Read the model definition and answer for the solid it produces. Units are mm, in the model's axes. A direction names the side the tool comes from. Coordinates: 2 decimals unless noted, no trailing zeros. Loops run counter-clockwise (first coordinate to the right, second up) from the corner with the lowest first, then second, coordinate; pieces in that order, holes last. Notation, with made-up numbers: (47.5, -28.5) - (81.5, -28.5) arc R6 ccw to (81.5, -20.5) - close; hole circle Ø9 at (82.5, 69). An arc over 180 degrees is marked (long way). One line per item, written item: value. Start each with the question number.
from build123d import *

# Parameters (mm, degrees)
SKETCH1_W           = 66.5
SKETCH1_H           = 180
BOSS_EXTRUDE1_DEPTH = 180
SKETCH3_W           = 160
SKETCH3_H           = 160
CUT_EXTRUDE1_DEPTH  = 180
SKETCH8_W           = 66.5
SKETCH8_H           = 40
BOSS_EXTRUDE2_DEPTH = 5
SKETCH10_W          = 66.5
SKETCH10_H          = 40
BOSS_EXTRUDE3_DEPTH = 5
SKETCH5_R           = 14
CUT_EXTRUDE3_DEPTH  = 10
SKETCH7_R           = 14
CUT_EXTRUDE4_DEPTH  = 10
CUT_EXTRUDE5_DEPTH  = 5
CUT_EXTRUDE6_START  = -5
CUT_EXTRUDE6_DEPTH  = 5
SKETCH12_W          = 66.5
SKETCH12_H          = 40
BOSS_EXTRUDE8_DEPTH = 5
SKETCH15_R          = 14
CUT_EXTRUDE7_DEPTH  = 200
SKETCH16_W          = 66.5
SKETCH16_H          = 40
BOSS_EXTRUDE9_DEPTH = 5
FILLET1_R           = 10
FILLET2_R           = 10


with BuildPart() as part:
    # Sketch1 → Boss-Extrude1 (new body)
    with BuildSketch(Plane.XY):
        with Locations((33.25, 90)):
            Rectangle(SKETCH1_W, SKETCH1_H)
    extrude(amount=BOSS_EXTRUDE1_DEPTH)

    # Sketch3 → Cut-Extrude1 (cut)
    with BuildSketch(Plane.ZY):
        with Locations((90, 90)):
            Rectangle(SKETCH3_W, SKETCH3_H)
    extrude(amount=-CUT_EXTRUDE1_DEPTH, mode=Mode.SUBTRACT)

    # Sketch8 → Boss-Extrude2 (add)
    with BuildSketch(Plane.XY.offset(10)):
        with Locations((33.25, 150)):
            Rectangle(SKETCH8_W, SKETCH8_H)
    extrude(amount=BOSS_EXTRUDE2_DEPTH)

    # Sketch10 → Boss-Extrude3 (add)
    with BuildSketch(Plane(origin=(0, 0, 170), x_dir=(-1, 0, 0), z_dir=(0, 0, -1))):
        with Locations((-33.25, 150)):
            Rectangle(SKETCH10_W, SKETCH10_H)
    extrude(amount=BOSS_EXTRUDE3_DEPTH)

    # Sketch5 → Cut-Extrude3 (cut)
    with BuildSketch(Plane(origin=(0, 180, 0), x_dir=(1, 0, 0), z_dir=(0, 1, 0))):
        with Locations(Location((49.5, -90, 0), (0, 0, 270))):
            Circle(SKETCH5_R)
    extrude(amount=-CUT_EXTRUDE3_DEPTH, mode=Mode.SUBTRACT)

    # Sketch7 → Cut-Extrude4 (cut)
    with BuildSketch(Plane.XZ):
        with Locations(Location((49.5, 50, 0), (0, 0, 270))):
            Circle(SKETCH7_R)
        with Locations(Location((49.5, 130, 0), (0, 0, 270))):
            Circle(SKETCH7_R)
    extrude(amount=-CUT_EXTRUDE4_DEPTH, mode=Mode.SUBTRACT)

    # Sketch9 → Cut-Extrude5 (cut)
    with BuildSketch(Plane.XY.offset(15)):
        with BuildLine():
            Line((60.5, 164.5), (7.5, 164.5))
            ThreePointArc((7.5, 164.5), (5.378679656, 163.621320344), (4.5, 161.5))
            Line((4.5, 161.5), (4.5, 138.5))
            ThreePointArc((4.5, 138.5), (5.378679656, 136.378679656), (7.5, 135.5))
            Line((7.5, 135.5), (60.5, 135.5))
            ThreePointArc((60.5, 135.5), (62.621320344, 136.378679656), (63.5, 138.5))
            Line((63.5, 138.5), (63.5, 161.5))
            ThreePointArc((63.5, 161.5), (62.621320344, 163.621320344), (60.5, 164.5))
        make_face()
    extrude(amount=-CUT_EXTRUDE5_DEPTH, mode=Mode.SUBTRACT)

    # Sketch11 → Cut-Extrude6 (cut)
    with BuildSketch(Plane(origin=(0, 0, 165), x_dir=(-1, 0, 0), z_dir=(0, 0, -1)).offset(CUT_EXTRUDE6_START)):
        with BuildLine():
            Line((-60.5, 164.5), (-7, 164.5))
            ThreePointArc((-7, 164.5), (-4.878679656, 163.621320344), (-4, 161.5))
            Line((-4, 161.5), (-4, 138.5))
            ThreePointArc((-4, 138.5), (-4.878679656, 136.378679656), (-7, 135.5))
            Line((-7, 135.5), (-60.5, 135.5))
            ThreePointArc((-60.5, 135.5), (-62.621320344, 136.378679656), (-63.5, 138.5))
            Line((-63.5, 138.5), (-63.5, 161.5))
            ThreePointArc((-63.5, 161.5), (-62.621320344, 163.621320344), (-60.5, 164.5))
        make_face()
    extrude(amount=CUT_EXTRUDE6_DEPTH, mode=Mode.SUBTRACT)

    # Sketch12 → Boss-Extrude8 (add)
    with BuildSketch(Plane.XZ.offset(-170)):
        with Locations((33.25, 89.833476808)):
            Rectangle(SKETCH12_W, SKETCH12_H)
        with BuildLine():
            Line((60.5, 75.333476808), (7, 75.333476808))
            ThreePointArc((7, 75.333476808), (4.878679656, 76.212156465), (4, 78.333476808))
            Line((4, 78.333476808), (4, 101.333476808))
            ThreePointArc((4, 101.333476808), (4.878679656, 103.454797152), (7, 104.333476808))
            Line((7, 104.333476808), (60.5, 104.333476808))
            ThreePointArc((60.5, 104.333476808), (62.621320344, 103.454797152), (63.5, 101.333476808))
            Line((63.5, 101.333476808), (63.5, 78.333476808))
            ThreePointArc((63.5, 78.333476808), (62.621320344, 76.212156465), (60.5, 75.333476808))
        make_face(mode=Mode.SUBTRACT)
    extrude(amount=BOSS_EXTRUDE8_DEPTH)

    # Sketch15 → Cut-Extrude7 (cut)
    with BuildSketch(Plane(origin=(0, 0, 0), x_dir=(-1, 0, 0), z_dir=(0, 0, -1))):
        with Locations((-17, 150)):
            Circle(SKETCH15_R)
    extrude(amount=-CUT_EXTRUDE7_DEPTH, mode=Mode.SUBTRACT)

    # Sketch16 → Boss-Extrude9 (add)
    # profile 1 of 2: a face of its own
    with BuildSketch(Plane(origin=(0, 10, 0), x_dir=(1, 0, 0), z_dir=(0, 1, 0))):
        with Locations((33.25, -50)):
            Rectangle(SKETCH16_W, SKETCH16_H)
        with BuildLine():
            Line((63.5, -38.5), (63.5, -61.5))
            ThreePointArc((63.5, -61.5), (62.621320344, -63.621320344), (60.5, -64.5))
            Line((60.5, -64.5), (7, -64.5))
            ThreePointArc((7, -64.5), (4.878679656, -63.621320344), (4, -61.5))
            Line((4, -61.5), (4, -38.5))
            ThreePointArc((4, -38.5), (4.878679656, -36.378679656), (7, -35.5))
            Line((7, -35.5), (60.5, -35.5))
            ThreePointArc((60.5, -35.5), (62.621320344, -36.378679656), (63.5, -38.5))
        make_face(mode=Mode.SUBTRACT)
    # profile 2 of 2: a face of its own
    with BuildSketch(Plane(origin=(0, 10, 0), x_dir=(1, 0, 0), z_dir=(0, 1, 0))):
        with Locations((33.25, -130)):
            Rectangle(SKETCH16_W, SKETCH16_H)
        with BuildLine():
            Line((63.5, -141.5), (63.5, -118.5))
            ThreePointArc((63.5, -118.5), (62.621320344, -116.378679656), (60.5, -115.5))
            Line((60.5, -115.5), (7, -115.5))
            ThreePointArc((7, -115.5), (4.878679656, -116.378679656), (4, -118.5))
            Line((4, -118.5), (4, -141.5))
            ThreePointArc((4, -141.5), (4.878679656, -143.621320344), (7, -144.5))
            Line((7, -144.5), (60.5, -144.5))
            ThreePointArc((60.5, -144.5), (62.621320344, -143.621320344), (63.5, -141.5))
        make_face(mode=Mode.SUBTRACT)
    extrude(amount=BOSS_EXTRUDE9_DEPTH)

    # Fillet1
    fillet1_edges = [part.edges().sort_by_distance(p)[0] for p in [
        (33.25, 180, 0),
        (33.25, 0, 0),
    ]]
    fillet(fillet1_edges, radius=FILLET1_R)

    # Fillet2
    fillet2_edges = [part.edges().sort_by_distance(p)[0] for p in [
        (33.25, 180, 180),
        (33.25, 0, 180),
    ]]
    fillet(fillet2_edges, radius=FILLET2_R)


solid = part.part
1) Section B-B, the plane y = 150 is taken. Determine the outline of the cut face in (x, z).
2) Section A-A, the plane y = 54 is taken. Determine the outline of the cut face in (x, z).
3) Straight lines are drawn through the part: L1, parallel to Y at x = 19.5, z = 74; L2, parallel to Z at x = 36.5, y = 82.5. For each, find the intervals that lie inside material, in ascending order.
4) Flat-ended cylindrical pins translate along their axes: P1, Ø2.5, axis at y = 146, z = 12.5, coming from the -X side; P2, Ø17, axis at x = 49.5, z = 50, coming from the -Y side. Find the tip coordinate at first contact, or state that the pin passes through.
5) Determine the mould class of faces 4 (the flat face through (33, 69, 10)), 5 (the cylindrical face through (33.72, 2.85, 3.01)), 6 (the cylindrical face through (33.72, 177.15, 176.99)) for opening direction Z: released by +Z, released by -Z, zero draft, split by the parting line, or undercut.
6) Section C-C, the plane x = 49.5 is taken. State how many separate pieces and enclosed holes the cut face has, and give its area (3 significant figures).
7) For faces 1 (the flat face through (33, 69, 170)), 2 (the flat face through (4.5, 141, 13)), 3 (the flat face through (33, 91, 180)), determine the directions among +Z, -Z, +X, -X, +Y, -Y from which every point of the face is accessible in a straight line to the end or side of a thin tool.
Answer below:
1. outline: (0, 0) - (3, 0) - (3, 15) - (0, 15) - close; (0, 165) - (3, 165) - (3, 180) - (0, 180) - close; (31, 0) - (66.5, 0) - (66.5, 15) - (63.5, 15) - (63.5, 10) - (31, 10) - close; (31, 170) - (63.5, 170) - (63.5, 165) - (66.5, 165) - (66.5, 180) - (31, 180) - close
2. outline: (0, 0) - (66.5, 0) - (66.5, 10) - (0, 10) - close; (0, 170) - (66.5, 170) - (66.5, 180) - (0, 180) - close
3. L1: 0 to 10, 165 to 180
3. L2: 0 to 10, 170 to 180
4. P1: x = 0
4. P2: y = 170
5. face 4: undercut
5. face 5: released by -Z
5. face 6: released by +Z
6. separate pieces: 3
6. enclosed holes: 0
6. area: 6,150 mm2
7. face 1: +X, -X
7. face 2: none
7. face 3: +Z, +X, -X, +Y, -Y
